from build123d import *

# Parameters (mm, degrees)
SKETCH1_W           = 9
SKETCH1_H           = 11
BASE_EXTRUDE_DEPTH  = 3.5
BOSS_EXTRUDE1_DEPTH = 9.9
SKETCH3_R           = 3.2
CUT_EXTRUDE1_DEPTH  = 9.144
SKETCH4_R           = 1
EXTRUDE1_DEPTH      = 7.804
FILLET1_R           = 0.5
BOSS_EXTRUDE2_DEPTH = 1
SKETCH22_W          = 0.413257786
SKETCH22_H          = 0.581135983
BOSS_EXTRUDE3_DEPTH = 0.4
SKETCH23_R          = 0.5
SKETCH23_R_2        = 0.375
BOSS_EXTRUDE4_DEPTH = 0.9
SKETCH24_W          = 2.2
SKETCH24_H          = 0.4
SKETCH24_H_2        = 0.25
BOSS_EXTRUDE5_DEPTH = 4.4
SKETCH5_R           = 0.75
EXTRUDE2_DEPTH      = 0.2
SKETCH25_R          = 0.5
CUT_EXTRUDE5_DEPTH  = 12.2
SKETCH26_R          = 1.235253259
BOSS_EXTRUDE6_DEPTH = 0.3
FILLET2_R           = 0.5
SKETCH28_W          = 8.199907687
SKETCH28_H          = 3.89034232
CUT_EXTRUDE6_DEPTH  = 1.75
BOSS_EXTRUDE7_DEPTH = 1.5


with BuildPart() as part:
    # Sketch1 → Base-Extrude (new body)
    with BuildSketch(Plane.XY):
        with Locations((0, 5.5)):
            Rectangle(SKETCH1_W, SKETCH1_H)
    extrude(amount=-BASE_EXTRUDE_DEPTH)

    # Sketch2 → Boss-Extrude1 (add)
    with BuildSketch(Plane(origin=(0, 0, -3.5), x_dir=(-1, 0, 0), z_dir=(0, 0, -1))):
        with BuildLine():
            Line((-4.5, 0), (-4.5, 6.4))
            Line((-4.5, 6.4), (-4.3, 6.4))
            ThreePointArc((-4.3, 6.4), (0, 10.7), (4.3, 6.4))
            Line((4.3, 6.4), (4.5, 6.4))
            Line((4.5, 6.4), (4.5, 0))
            Line((4.5, 0), (-4.5, 0))
        make_face()
    extrude(amount=BOSS_EXTRUDE1_DEPTH)

    # Sketch3 → Cut-Extrude1 (cut)
    with BuildSketch(Plane.XY):
        with Locations((0, 6.4)):
            Circle(SKETCH3_R)
    extrude(amount=-CUT_EXTRUDE1_DEPTH, mode=Mode.SUBTRACT)

    # Sketch4 → Extrude1 (add)
    with BuildSketch(Plane.XY.offset(-9.144)):
        with Locations((0, 6.4)):
            Circle(SKETCH4_R)
    extrude(amount=EXTRUDE1_DEPTH)

    # Fillet1
    fillet1_edges = [part.edges().sort_by_distance(p)[0] for p in [
        (-1, 6.4, -1.34),
    ]]
    fillet(fillet1_edges, radius=FILLET1_R)

    # Sketch21 → Boss-Extrude2 (add)
    with BuildSketch(Plane(origin=(0, 0, -13.4), x_dir=(-1, 0, 0), z_dir=(0, 0, -1))):
        with BuildLine():
            Line((2.531952195, 9.496646264), (4.5, 9.496646264))
            Line((4.5, 9.496646264), (4.5, 6.4))
            Line((4.5, 6.4), (4.5, 0))
            Line((4.5, 0), (-4.5, 0))
            Line((-4.5, 0), (-4.5, 6.4))
            Line((-4.5, 6.4), (-4.5, 9.496646264))
            Line((-4.5, 9.496646264), (-2.531952195, 9.496646264))
            ThreePointArc((-2.531952195, 9.496646264), (0, 10.4), (2.531952195, 9.496646264))
        make_face()
    extrude(amount=BOSS_EXTRUDE2_DEPTH)

    # Sketch22 → Boss-Extrude3 (add)
    with BuildSketch(Plane(origin=(0, 0, -14.4), x_dir=(-1, 0, 0), z_dir=(0, 0, -1))):
        with BuildLine():
            Line((2.55496541, 7.9), (4.9, 7.9))
            Line((4.9, 7.9), (4.9, 4.9))
            Line((4.9, 4.9), (2.55496541, 4.9))
            Line((2.55496541, 4.9), (2.55496541, 4.366018911))
            Line((2.55496541, 4.366018911), (0, 4.366018911))
            ThreePointArc((0, 4.366018911), (-2.033981089, 6.4), (0, 8.433981089))
            Line((0, 8.433981089), (2.55496541, 8.433981089))
            Line((2.55496541, 8.433981089), (2.55496541, 7.9))
        make_face()
        with Locations((2.522410809, 6.417062755)):
            Rectangle(SKETCH22_W, SKETCH22_H, mode=Mode.SUBTRACT)
    extrude(amount=BOSS_EXTRUDE3_DEPTH)

    # Sketch23 → Boss-Extrude4 (add)
    with BuildSketch(Plane(origin=(0, 0, -14.4), x_dir=(-1, 0, 0), z_dir=(0, 0, -1))):
        with Locations((-3.5, 0.8)):
            Circle(SKETCH23_R)
        with Locations((3.5, 0.8)):
            Circle(SKETCH23_R)
        with Locations((-3.5, 8.6)):
            Circle(SKETCH23_R)
        with Locations((3.5, 8.6)):
            Circle(SKETCH23_R_2)
    extrude(amount=BOSS_EXTRUDE4_DEPTH)

    # Sketch24 → Boss-Extrude5 (add)
    with BuildSketch(Plane(origin=(0, 0, -14.4), x_dir=(-1, 0, 0), z_dir=(0, 0, -1))):
        with Locations((-1.4, 3.6)):
            Rectangle(SKETCH24_W, SKETCH24_H)
        with Locations((1.4, 0.8)):
            Rectangle(SKETCH24_W, SKETCH24_H_2)
    extrude(amount=BOSS_EXTRUDE5_DEPTH)

    # Sketch5 → Extrude2 (add, symmetric)
    with BuildSketch(Plane(origin=(-4.9, 0, 0), x_dir=(0, 0, -1), z_dir=(1, 0, 0))):
        with BuildLine():
            Line((14.4, 7.9), (17.3, 7.9))
            ThreePointArc((17.3, 7.9), (18.8, 6.4), (17.3, 4.9))
            Line((17.3, 4.9), (14.4, 4.9))
            Line((14.4, 4.9), (14.4, 7.9))
        make_face()
        with Locations((17.3, 6.4)):
            Circle(SKETCH5_R, mode=Mode.SUBTRACT)
    extrude(amount=EXTRUDE2_DEPTH, both=True)

    # Sketch25 → Cut-Extrude5 (cut)
    with BuildSketch(Plane(origin=(0, 3.8, 0), x_dir=(1, 0, 0), z_dir=(0, 1, 0))):
        with Locations((-1.4, 17.7)):
            Circle(SKETCH25_R)
        with Locations((1.4, 17.7)):
            Circle(SKETCH25_R)
        with BuildLine():
            Line((0.3, 17.7), (0.3, 18.8))
            Line((0.3, 18.8), (1.814838084, 19.127754717))
            Line((1.814838084, 19.127754717), (2.5, 18.8))
            Line((2.5, 18.8), (2.5, 17.7))
            ThreePointArc((2.5, 17.7), (1.4, 18.8), (0.3, 17.7))
        make_face()
        with BuildLine():
            Line((-2.5, 17.7), (-2.5, 18.8))
            Line((-2.5, 18.8), (-1.388936506, 19.127754717))
            Line((-1.388936506, 19.127754717), (-0.3, 18.8))
            Line((-0.3, 18.8), (-0.3, 17.7))
            ThreePointArc((-0.3, 17.7), (-1.4, 18.8), (-2.5, 17.7))
        make_face()
    extrude(amount=-CUT_EXTRUDE5_DEPTH, mode=Mode.SUBTRACT)

    # Sketch26 → Boss-Extrude6 (add)
    with BuildSketch(Plane(origin=(0, 0, -14.8), x_dir=(-1, 0, 0), z_dir=(0, 0, -1))):
        with Locations((0.197894438, 6.4)):
            Circle(SKETCH26_R)
    extrude(amount=BOSS_EXTRUDE6_DEPTH)

    # Fillet2
    fillet2_edges = [part.edges().sort_by_distance(p)[0] for p in [
        (0, 11, 0),
        (4.5, 5.5, 0),
        (0, 0, 0),
        (-4.5, 5.5, 0),
        (4.5, 8.7, -3.5),
        (4.5, 0, -7.2),
        (-4.5, 0, -7.2),
        (4.5, 11, -1.75),
        (0, 11, -3.5),
        (-4.5, 8.7, -3.5),
        (-4.5, 11, -1.75),
    ]]
    fillet(fillet2_edges, radius=FILLET2_R)

    # Sketch28 → Cut-Extrude6 (cut, symmetric)
    with BuildSketch(Plane(origin=(0, 0, 0), x_dir=(0, 0, -1), z_dir=(1, 0, 0))):
        with Locations((5.030081863, 3.009711686)):
            Rectangle(SKETCH28_W, SKETCH28_H)
    extrude(amount=CUT_EXTRUDE6_DEPTH, both=True, mode=Mode.SUBTRACT)

    # Sketch27 → Boss-Extrude7 (add, symmetric)
    with BuildSketch(Plane(origin=(0, 0, 0), x_dir=(0, 0, -1), z_dir=(1, 0, 0))):
        with BuildLine():
            Line((0.855128644, 3.105078739), (2.30673576, 3.9461551))
            ThreePointArc((2.30673576, 3.9461551), (4.216159937, 4.339068854), (6.125584114, 3.9461551))
            Line((6.125584114, 3.9461551), (9.059931405, 2.68512141))
            Line((9.059931405, 2.68512141), (8.9414814, 2.409495584))
            Line((8.9414814, 2.409495584), (6.007134108, 3.670529274))
            ThreePointArc((6.007134108, 3.670529274), (4.224971911, 4.039060295), (2.441391305, 3.677456327))
            Line((2.441391305, 3.677456327), (1.005529549, 2.845502993))
            Line((1.005529549, 2.845502993), (0.855128644, 3.105078739))
        make_face()
    extrude(amount=BOSS_EXTRUDE7_DEPTH, both=True)


solid = part.part
Check sheet for the modelled part. Datum: model origin and axes. Units: mm. A direction names the side the tool comes from. Coordinates: 2 decimals unless noted, no trailing zeros. Write each loop counter-clockwise with the first axis right and the second up, starting at its lowest first coordinate (ties: lowest second). Pieces come first, ordered by that corner, then holes.
Item 1: Cross-section at C-C on x = -3.5. Record the boundary of the cut face in (y, z) (3 decimals), then the cut area to 3 significant figures.
Numbers:
outline: (0, -14.4) - (0.3, -14.4) - (0.3, -15.3) - (1.3, -15.3) - (1.3, -14.4) - (4.9, -14.4) - (4.9, -14.8) - (7.9, -14.8) - (7.9, -14.4) - (8.225, -14.4) - (8.225, -15.3) - (8.975, -15.3) - (8.975, -14.4) - (9.497, -14.4) - (9.497, -13.4) - (8.898, -13.4) - (8.898, -3.5) - (10.5, -3.5) arc R0.5 ccw to (11, -3) - (11, -0.5) arc R0.5 ccw to (10.5, 0) - (0.5, 0) arc R0.5 ccw to (0, -0.5) - close
area: 139 mm2
Item 2: Cross-section at A-A on z = -7.5. Record the boundary of the cut face in (x, y), then the cut area to 3 significant figures.
Numbers:
outline: (-4.5, 0.5) arc R0.5 ccw to (-4, 0) - (4, 0) arc R0.5 ccw to (4.5, 0.5) - (4.5, 6.4) - (4.3, 6.4) arc R4.3 ccw to (-4.3, 6.4) - (-4.5, 6.4) - close; (-1.5, 3.03) - (1.5, 3.03) - (1.5, 3.36) - (-1.5, 3.36) - close; circle Ø2 at (0, 6.4); hole (-1.75, 1.06) - (1.75, 1.06) - (1.75, 3.72) arc R3.2 ccw (long way) to (-1.75, 3.72) - close
area: 50.4 mm2
Item 3: Access from +Z, -Z, +X, -X, +Y, -Y to the whole of each face (thin tool, end or side, straight path). Record for faces 1 (the face through (-1, 0.925, -17)), 2 (the face through (-0.217, 5.424, -5.543)), 3 (the face through (-1.75, 2, -5)), 4 (the face through (1, 3.4, -17)).
Numbers:
face 1: -Z
face 2: +Z
face 3: none
face 4: -Z, +X, -X, -Y
Item 4: Mould release check, pull along Z, two halves, no side actions. Record for faces 5 (the face through (3.5, 0.8, -15.3)), 6 (the face through (0, 11, -2)), 7 (the face through (0.021, 3.267, -1.734)): released by +Z, released by -Z, zero draft, split by the parting line, or undercut.
Numbers:
face 5: released by -Z
face 6: zero draft
face 7: undercut
Item 5: Depth check by flat-ended pin: pin 1 Ø0.5 at (x, y) = (3.5, 0.5) entering from -Z; pin 2 Ø1.1 at (x, z) = (3.5, -14) entering from +Y; pin 3 Ø0.7 at (x, z) = (-1, -15.5) entering from +Y (3 decimals). Enter the tip coordinate at first touch or a pass-through.
Numbers:
pin 1: stops at z = -15.3
pin 2: stops at y = 9.5
pin 3: stops at y = 0.925
Item 6: Cross-section at B-B on y = 2. Record the boundary of the cut face in (x, z).
Numbers:
outline: (-4.5, -14.4) - (4.5, -14.4) - (4.5, -0.5) arc R0.5 ccw to (4, 0) - (-4, 0) arc R0.5 ccw to (-4.5, -0.5) - close; hole (-1.75, -9.13) - (1.75, -9.13) - (1.75, -0.93) - (-1.75, -0.93) - close
Item 7: Cross-section at D-D on z = -10.25. Record the boundary of the cut face in (x, y), then the cut area to 3 significant figures.
Numbers:
outline: (-4.5, 0.5) arc R0.5 ccw to (-4, 0) - (4, 0) arc R0.5 ccw to (4.5, 0.5) - (4.5, 6.4) - (4.3, 6.4) arc R4.3 ccw to (-4.3, 6.4) - (-4.5, 6.4) - close
area: 86.5 mm2
Item 8: Scan lines: probe 1 along Y at (x, z) = (3.5, -15.25); probe 2 along X at (y, z) = (2.75, -4); probe 3 along Y at (x, z) = (0, -8.25). Record each from-to range of solid material in increasing order.
Numbers:
probe 1: y = 0.3 to 1.3, 8.1 to 9.1
probe 2: x = -4.5 to -1.75, 1.75 to 4.5
probe 3: y = 0 to 1.06, 2.71 to 3.03, 5.4 to 7.4, 9.6 to 10.7
